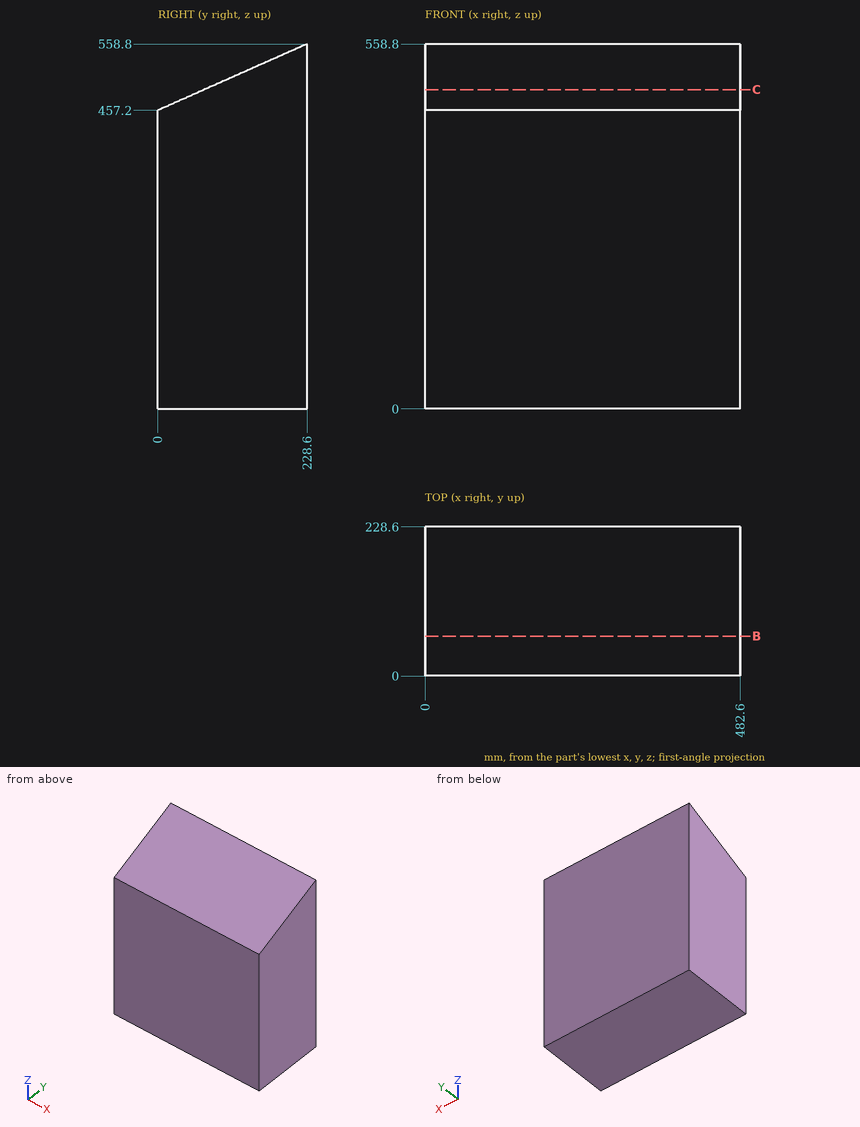
Check sheet for the drawn part. Datum: minimum x, y, z corner. Units: mm. Round coordinates to 2 decimals unless told otherwise and drop trailing zeros. Order: outer loops, then holes, each group sorted by start corner. A loop starts at its lowest first (then second) coordinate and runs counter-clockwise, first axis right, second up. Notation, with made-up numbers: (63, 16.5) -> (80, 16.5) arc R26 cw to (80, 51.5) -> close; hole circle Ø11 at (44.5, 76). An arc over 180 degrees is marked (long way). Use CSV: the item, a comma, the result in double quotes.
(1) Material ranges on line 1 along Z through (x, y) = (180, 36.5); line 2 along Z through (x, y) = (132, 149); line 3 along Y through (x, z) = (248, 514.5) (3 decimals), recorded low to high. Write a range as from..to.
Worked out:
line 1,"0..473.42"
line 2,"0..523.42"
line 3,"128.925..228.6"
(2) Cross-section at C-C (z = 489). Record the boundary of the cut face in (x, y), and give its area (3 significant figures).
Worked out:
outline,"(0, 71.55) -> (482.6, 71.55) -> (482.6, 228.6) -> (0, 228.6) -> close"
area,"75,800 mm²"
(3) Cross-section at B-B (y = 61). Record the boundary of the cut face in (x, z).
Worked out:
outline,"(0, 0) -> (482.6, 0) -> (482.6, 484.31) -> (0, 484.31) -> close"
(4) Depth check by flat-ended pin: pin 1 (1.5 mm diameter, centred on x = 220, y = 167.5, fed in from +Z). Enter the tip coordinate at first touch or a pass-through.
Worked out:
pin 1,"z = 531.98"
